Source: CAD feature listing. Evaluate the final solid. Frame: model axes, mm. A direction names the side the tool comes from. Round coordinates to 2 decimals unless told otherwise and drop trailing zeros. Loops run counter-clockwise (first coordinate to the right, second up) from the corner with the lowest first, then second, coordinate; pieces in that order, holes last. Notation, with made-up numbers: M 8.25,24 L 21.25,24 A27 ccw 21.25,59 Z; hole C 44.25,48 d2. An arc over 180 degrees is marked long. One line per item, written item: value.
from build123d import *

# Parameters (mm, degrees)
SKETCH1_W           = 112
SKETCH1_H           = 75
BOSS_EXTRUDE1_DEPTH = 4.5
SKETCH2_R           = 2.55
SKETCH2_R_2         = 3.5
SKETCH2_W           = 10
SKETCH2_H           = 25
CUT_EXTRUDE1_DEPTH  = 135.867527597
FILLET1_R           = 5


with BuildPart() as part:
    # Sketch1 → Boss-Extrude1 (new body)
    with BuildSketch(Plane(origin=(0, 0, 0), x_dir=(1, 0, 0), z_dir=(0, 1, 0))):
        with Locations((56, 37.5)):
            Rectangle(SKETCH1_W, SKETCH1_H)
    extrude(amount=BOSS_EXTRUDE1_DEPTH)

    # Sketch2 → Cut-Extrude1 (cut, through all)
    with BuildSketch(Plane(origin=(0, 4.5, 0), x_dir=(1, 0, 0), z_dir=(0, 1, 0))):
        with Locations(Location((95.5, 16.5, 0), (0, 0, 270))):
            Circle(SKETCH2_R)
        with Locations(Location((16.5, 16.5, 0), (0, 0, 270))):
            Circle(SKETCH2_R)
        with Locations(Location((16.5, 59, 0), (0, 0, 270))):
            Circle(SKETCH2_R_2)
        with Locations(Location((95.5, 59, 0), (0, 0, 270))):
            Circle(SKETCH2_R_2)
        with Locations((5, 38)):
            Rectangle(SKETCH2_W, SKETCH2_H)
        with Locations((107, 38)):
            Rectangle(SKETCH2_W, SKETCH2_H)
    extrude(amount=-CUT_EXTRUDE1_DEPTH, mode=Mode.SUBTRACT)

    # Fillet1
    fillet1_edges = [part.edges().sort_by_distance(p)[0] for p in [
        (112, 2.25, -50.5),
        (112, 2.25, -25.5),
        (0, 2.25, -25.5),
        (0, 2.25, -50.5),
        (0, 2.25, -75),
        (112, 2.25, -75),
        (112, 2.25, 0),
        (0, 2.25, 0),
    ]]
    fillet(fillet1_edges, radius=FILLET1_R)


solid = part.part
1. Ray query, line 1 (X direction, y = 1.3, z = -59); line 2 (X direction, y = 2.25, z = -58); line 3 (X direction, y = 3.8, z = -47). Return the intervals inside material, ascending. Write a range as [from, to].
Report:
line 1: x = [0, 13], [20, 92], [99, 112]
line 2: x = [0, 13.15], [19.85, 92.15], [98.85, 112]
line 3: x = [10, 102]
2. Section query A-A (z = -59). Return the cut outline in (x, y).
Report:
outline: M 0,0 L 13,0 L 13,4.5 L 0,4.5 Z; M 20,0 L 92,0 L 92,4.5 L 20,4.5 Z; M 99,0 L 112,0 L 112,4.5 L 99,4.5 Z
3. Pin query (flat end, axial travel): pin 1 (2 mm diameter, centred on y = 2.5, z = -33.5, fed in from +X); pin 2 (3 mm diameter, centred on x = 95.5, z = -16.5, fed in from -Y). Return the tip coordinate at first contact, or that it passes through.
Report:
pin 1: stops at x = 102
pin 2: passes through
4. Section query B-B (x = 16.5). Return the cut outline in (y, z).
Report:
outline: M 0,-75 L 4.5,-75 L 4.5,-62.5 L 0,-62.5 Z; M 0,-55.5 L 4.5,-55.5 L 4.5,-19.05 L 0,-19.05 Z; M 0,-13.95 L 4.5,-13.95 L 4.5,0 L 0,0 Z
5. Section query D-D (z = -33). Return the cut outline in (x, y), and give its area (3 significant figures).
Report:
outline: M 10,0 L 102,0 L 102,4.5 L 10,4.5 Z
area: 414 mm2
6. Reachability of faces 1 (the face through (110.5, 2.22, -24.07)), 2 (the face through (10, 2, -38)), 3 (the face through (0, 2, -63)) from +Z, -Z, +X, -X, +Y, -Y: full face, straight path, thin tool, end or side. Return the list, or none.
Report:
face 1: +X, +Y, -Y
face 2: -X, +Y, -Y
face 3: +Z, -Z, -X, +Y, -Y
7. Section query C-C (y = 3). Return the cut outline in (x, z), and give its area (3 significant figures).
Report:
outline: M 0,-70 A5 ccw 5,-75 L 107,-75 A5 ccw 112,-70 L 112,-55.5 A5 ccw 107,-50.5 L 102,-50.5 L 102,-25.5 L 107,-25.5 A5 ccw 112,-20.5 L 112,-5 A5 ccw 107,0 L 5,0 A5 ccw 0,-5 L 0,-20.5 A5 ccw 5,-25.5 L 10,-25.5 L 10,-50.5 L 5,-50.5 A5 ccw 0,-55.5 Z; hole C 16.5,-59 d7; hole C 16.5,-16.5 d5.1; hole C 95.5,-59 d7; hole C 95.5,-16.5 d5.1
area: 7,740 mm2
